Autodesk Inventor part; units mm, degrees
ref_plane "YZ Plane" through (0, 0, 0) normal (1, 0, 0) x (0, 1, 0)
ref_plane "XZ Plane" through (0, 0, 0) normal (0, 1, 0) x (-1, 0, 0)
ref_plane "XY Plane" through (0, 0, 0) normal (0, 0, 1) x (1, 0, 0)
sketch "草图1" plane through (0, 0, 0) normal (1, 0, 0) x (0, 1, 0)
  circle A0 centre (4.0723, -9.46) radius 2.95
  line L0 (16.324, 0) -> (-17.1797, 0)
  line L1 (1.1223, -9.46) -> (1.1223, 0)
  line L2 (6.1223, 0) -> (6.1223, -7.3387)
  circle A1 centre (4.0723, 9.46) radius 1.2
  line L3 (6.1223, 0) -> (6.1223, 11)
  line L4 (1.1223, 0) -> (1.1223, 12)
  line L5 (1.1223, 12) -> (5.1223, 12)
  circle A2 centre (4.0723, -9.46) radius 1.1
  line L6 (5.1223, 12) -> (6.1223, 11)
  line L7 (4.0723, -12.41) -> (1.1223, -12.41)
  line L8 (1.1223, -12.41) -> (1.1223, -9.46)
  point P0 (0, 0)
  dimension "d0" = 5.9
  dimension "d2" = 18.92
  dimension "d3" = 2.4
  dimension "d4" = 5
  dimension "d5" = 2.2
  dimension "d8" = 135
  dimension "d9" = 24
  dimension "d10" = 1
extrude "拉伸1" add sketch "草图1" along normal blind 8
sketch "草图2" plane through (8, 0, 0) normal (1, 0, 0) x (0, 0, -1)
  line L0 (-11, 6.1223) -> (-12, 5.1223)
  line L1 (-12, 5.1223) -> (-12, 1.1223)
  line L2 (-12, 1.1223) -> (12.41, 1.1223)
  line L3 (12.41, 1.1223) -> (12.41, 4.0723)
  arc A0 (12.41, 4.0723) -> (7.3387, 6.1223) centre (9.46, 4.0723) ccw
  line L4 (7.3387, 6.1223) -> (-11, 6.1223)
  circle A1 centre (9.46, 4.0723) radius 1.1
  circle A2 centre (-9.46, 4.0723) radius 1.2
  line L5 (7.3387, 6.1223) -> (-11, 6.1223)
  line L6 (5.46, 6.1223) -> (5.46, 1.1223)
  point P0 (0, 0)
  point P1 (5.46, 3.6223)
  dimension "d11" = 4
extrude "拉伸2" add sketch "草图2" along normal blind 25 contours L4 L6 L2 L1 L0
sketch "草图3" plane through (33, 0, 0) normal (1, 0, 0) x (0, 0, -1)
  line L0 (-12, 1.1223) -> (5.46, 1.1223)
  line L1 (5.46, 1.1223) -> (5.46, 6.1223)
  line L2 (5.46, 6.1223) -> (-11, 6.1223)
  line L3 (-11, 6.1223) -> (-12, 5.1223)
  line L4 (-12, 5.1223) -> (-12, 1.1223)
  circle A0 centre (-9.46, 4.0723) radius 1.2
  line L5 (-12, 1.1223) -> (12.41, 1.1223)
  line L6 (5.46, 1.1223) -> (12.41, 1.1223)
  line L7 (12.41, 1.1223) -> (12.41, 6.1223)
  line L8 (12.41, 6.1223) -> (5.46, 6.1223)
  circle A1 centre (9.46, 4.0723) radius 1.1
  arc A2 (12.41, 4.0723) -> (7.3387, 6.1223) centre (9.46, 4.0723) ccw
  point P0 (0, 0)
extrude "拉伸3" add sketch "草图3" along normal blind 5.9 contours L4 L3 L2 L1 L0 | L1 L8 A2 L7 L5 | A2 L8 L7
sketch "草图4" plane through (38.9, 0, 0) normal (1, 0, 0) x (0, 0, -1)
  circle A0 centre (9.46, 4.0723) radius 1.1
  circle A1 centre (9.46, 4.0723) radius 2.95
  line L0 (-12, 1.1223) -> (12.41, 1.1223)
  point P0 (0, 0)
  point P1 (8.9146, 1.1223)
  point P2 (9.46, 1.1223)
  dimension "d16" = 5.9
extrude "拉伸4" add sketch "草图4" along normal blind 6
chamfer "倒角1" distance 2 angle 45 1 edges at (20.5, 6.1223, -5.46)
chamfer "倒角2" distance 1 angle 45 1 edges at (19.45, 1.1223, 12)
chamfer "倒角3" distance 1 angle 45 1 edges at (20.5, 1.1223, -5.46)
sketch "草图5" plane through (0, 0, 0) normal (-1, 0, 0) x (0, 0, 1)
  line L0 (-7.3387, 6.1223) -> (11, 6.1223)
  line L1 (5.46, 6.1223) -> (5.46, 1.1223)
  line L2 (11, 1.1223) -> (-12.41, 1.1223)
  circle A0 centre (9.46, 4.0723) radius 1.2
  line L3 (12, 5.1223) -> (12, 2.1223)
  line L4 (11, 6.1223) -> (12, 5.1223)
  line L5 (12, 2.1223) -> (11, 1.1223)
  point P0 (0, 0)
  dimension "d28" = 4
extrude "拉伸5" cut sketch "草图5" against normal blind 8.2
sketch "草图6" plane through (38.9, 0, 0) normal (1, 0, 0) x (0, 0, -1)
  line L0 (-12, 5.1223) -> (-12, 2.1223)
  line L1 (-11, 6.1223) -> (-12, 5.1223)
  line L2 (-5.46, 6.1223) -> (-11, 6.1223)
  line L3 (-5.46, 1.1223) -> (-5.46, 6.1223)
  line L4 (-11, 1.1223) -> (-5.46, 1.1223)
  line L5 (-12, 2.1223) -> (-11, 1.1223)
  circle A0 centre (-9.46, 4.0723) radius 1.2
  point P0 (0, 0)
extrude "拉伸6" cut sketch "草图6" against normal blind 6.2
chamfer "倒角5" distance 2 angle 45 2 edges at (38.9, 3.6223, 5.46) (0, 3.6223, 5.46)
ref_plane "工作平面1" through (20.1, 0, 0) normal (1, 0, 0) x (0, 0, -1)
sketch "草图7" plane through (20.1, 0, 0) normal (1, 0, 0) x (0, 0, -1)
  line L0 (7.3387, 6.1223) -> (-3.46, 6.1223)
  line L1 (0.46, 6.1223) -> (-0.7743, 13.1223)
  line L2 (-0.7743, 13.1223) -> (-5.7743, 13.1223)
  line L3 (-5.7743, 13.1223) -> (-7.0086, 6.1223)
  line L4 (-7.0086, 6.1223) -> (0.46, 6.1223)
  point P0 (0, 0)
  point P1 (7.2697, 6.1223)
  point P2 (3.46, 6.1223)
  point P3 (-3.46, 6.1223)
  dimension "d40" = 80
  dimension "d41" = 80
  dimension "d42" = 5
  dimension "d43" = 3
  dimension "d44" = 7
extrude "拉伸7" add sketch "草图7" along normal blind 3.8
sketch "草图8" plane through (8.2, 2.1223, 12) normal (0, 0, 1) x (1, 0, 0)
  line L0 (11.9, 11) -> (15.7, 11)
  line L1 (11.9, 11) -> (11.9, 4)
  line L2 (12.3895, 11) -> (11.9, 4)
  line L3 (15.7, 11) -> (15.7, 4)
  line L4 (15.2105, 11) -> (15.7, 4)
  line L5 (11.9, 4) -> (15.7, 4)
  line L6 (15.7, 4) -> (11.9, 4)
  point P0 (-8.2, -2.1223)
  dimension "d47" = 86
  dimension "d48" = 86
extrude "拉伸8" cut sketch "草图8" against normal blind 100 contours L0 L2 L1 | L0 L3 L4
properties part number "履带片"
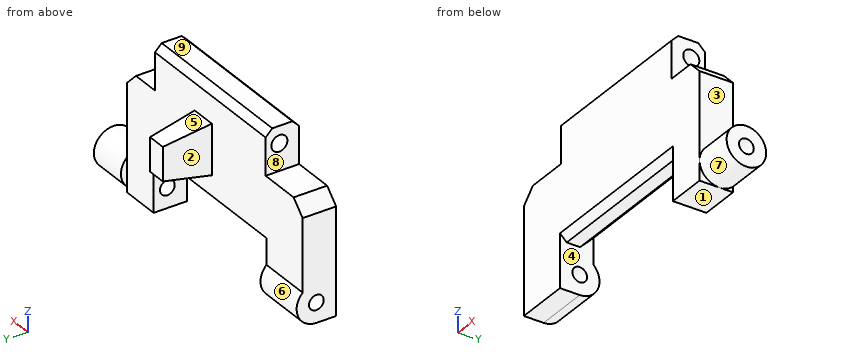
Design review of the part built by this model. Coordinates are the model's own, in mm. Face numbers are marked on the shaded views. A direction names the side the tool comes from. Give positions to 0.01 mm unless a question says otherwise; leave off trailing zeros. Order: outer loops, then holes, each group sorted by start corner. A loop starts at its lowest first (then second) coordinate and runs counter-clockwise, first axis right, second up. Notation, with made-up numbers: (10.5, 31) - (21.5, 31) arc R17 ccw to (21.5, 58) - close; hole circle Ø5 at (58, 63.5). An arc over 180 degrees is marked (long way). Use a Markdown table: item, result. Add a question column.
(1) Wall thickness on probe 1 along Y at (x, z) = (15, 9.46); probe 2 along Y at (x, z) = (2, -9.46); probe 3 along Y at (x, z) = (2, 4.25): over which ranges is each line inside the solid? List them lowest first. Write a range as [from, to].
(2) Add section D-D on x = 31.5. Give the boundary of the cut face in (y, z), then the cut area to 3 significant figures.
(3) Add section B-B on x = 21.5. Give the boundary of the cut face in (y, z), then the cut area to 3 significant figures.
(4) Mouldability with a two-part tool opening along X and no side actions: class the marked faces 1, 2, 3 and 4 as +X half, -X half, draft (parallel to the pull), parting line (faces both ways), or undercut.
(5) Machinability: for the marked faces 5, 6, 7, 8 and 9, which of the approach directions +Z, -Z, +X, -X, +Y, -Y give a long, thin tool a straight path to every point of the face, cutting with its end or side? Answer none if there is none.
(6) Add section A-A on z = 9.46. Give the boundary of the cut face in (x, y), then the cut area to 3 significant figures.
(7) Add section C-C on z = 1.5. Give the boundary of the cut face in (x, y), then the cut area to 3 significant figures.
(8) Clearance check with flat-ended pins moving along their axes: P1, Ø5, axis at y = 7, z = -2.5, coming from the -X side; P2, Ø4.5, axis at x = 35, y = 3.5, coming from the +Z side; P3, Ø0.6, axis at x = 25.5, y = 3.5, coming from the -Z side; P4, Ø10, axis at x = 32, z = 9, coming from the +Y side. State where each tip first meets the part, or that it passes through.
Report:
| question | item | result |
|---|---|---|
| 1 | probe 1 | y = [1.12, 2.87], [5.27, 6.12] |
| 1 | probe 2 | y = [1.12, 2.97], [5.17, 7.02] |
| 1 | probe 3 | y = [1.12, 6.12] |
| 2 | outline | (1.12, -4.46) - (2.12, -5.46) - (4.12, -5.46) - (6.12, -3.46) - (6.12, 11) - (5.12, 12) - (2.12, 12) - (1.12, 11) - close; hole circle Ø2.4 at (4.07, 9.46) |
| 2 | area | 79.3 mm² |
| 3 | outline | (1.12, -4.46) - (2.12, -5.46) - (4.12, -5.46) - (6.12, -3.46) - (6.12, -0.46) - (13.12, 0.77) - (13.12, 5.77) - (6.12, 7.01) - (6.12, 11) - (5.12, 12) - (2.12, 12) - (1.12, 11) - close; hole circle Ø2.4 at (4.07, 9.46) |
| 3 | area | 123 mm² |
| 4 | face 1 | draft |
| 4 | face 2 | -X half |
| 4 | face 3 | +X half |
| 4 | face 4 | undercut |
| 5 | face 5 | +Z, +X, -X, +Y |
| 5 | face 6 | -X, +Y |
| 5 | face 7 | +X |
| 5 | face 8 | +Z, -X, +Y, -Y |
| 5 | face 9 | +Z, +X, -X, +Y, -Y |
| 6 | outline | (8.2, 1.12) - (32.7, 1.12) - (32.7, 2.87) - (8.2, 2.87) - close; (8.2, 5.27) - (32.7, 5.27) - (32.7, 6.12) - (8.2, 6.12) - close |
| 6 | area | 63.7 mm² |
| 7 | outline | (0, 1.12) - (38.9, 1.12) - (38.9, 6.12) - (23.9, 6.12) - (23.41, 13.12) - (20.59, 13.12) - (20.1, 6.12) - (0, 6.12) - close |
| 7 | area | 218 mm² |
| 8 | P1 | stops at x = 0 |
| 8 | P2 | stops at z = 5.46 |
| 8 | P3 | stops at z = -5.46 |
| 8 | P4 | stops at y = 6.12 |
